Autodesk Inventor part; units mm, degrees
ref_plane "YZ Plane" through (0, 0, 0) normal (1, 0, 0) x (0, 1, 0)
ref_plane "XZ Plane" through (0, 0, 0) normal (0, 1, 0) x (-1, 0, 0)
ref_plane "XY Plane" through (0, 0, 0) normal (0, 0, 1) x (1, 0, 0)
sketch "Sketch1" plane through (0, 0, 0) normal (0, 1, 0) x (-1, 0, 0)
  circle A0 centre (0, 0) radius 6
  dimension "d0" = 12
extrude "Extrusion1" add sketch "Sketch1" along normal blind 1
fillet "Fillet1" radius 0.5 1 edges at (6, 0, 0)
sketch "Sketch2" plane through (0, 1, 0) normal (0, 1, 0) x (1, 0, 0)
  circle A0 centre (0, 0) radius 0.5
  dimension "d4" = 1
extrude "Extrusion2" cut sketch "Sketch2" against normal blind 1
sketch "Sketch3" plane through (0, 1, 0) normal (0, 1, 0) x (1, 0, 0)
  circle A0 centre (0, 0) radius 0.5
  circle A1 centre (0, 0) radius 5
  circle A2 centre (0, 0) radius 4
  dimension "d7" = 10
  dimension "d8" = 8
extrude "Extrusion3" add sketch "Sketch3" along normal blind 3 contours A1
chamfer "Chamfer1" distance 0.75 distance2 1.5 1 edges at (-4, 4, 0) measured on face at (4.5795, 4, 0.7179)
fillet "Fillet2" radius 0.2 1 edges at (-4.75, 4, 0)
fillet "Fillet3" radius 0.5 1 edges at (-4, 2.5, 0)
properties part number "tale"
Design review of the part built by this model. Coordinates are the model's own, in mm. Coordinates: 2 decimals unless noted, no trailing zeros. Write each loop counter-clockwise with the first axis right and the second up, starting at its lowest first coordinate (ties: lowest second). Pieces come first, ordered by that corner, then holes.
1) Mouldability with a two-part tool opening along X and no side actions: class faces 1 (the cylindrical face through (-0.108, 0.507, 0.488)), 2 (the flat face through (0, 0, -1)), 3 (the cylindrical face through (5.994, 0.746, -0.264)), 4 (the flat face through (0, 1, -1)) as +X half, -X half, draft (parallel to the pull), parting line (faces both ways), or undercut.
2) Add section A-A (y = 1.25). Write out the cut boundary in (x, z), plus the area to 3 significant figures.
3) To check wall thickness, follow L1, parallel to X at y = 1.45, z = 0; L2, parallel to Y at x = 4.5, z = 2.5. State the ranges of each line that lie inside material, in increasing order.
4) Insertion check: pin 1 (1.5 mm diameter, centred on y = 2, z = -1.5, fed in from -X); pin 2 (7 mm diameter, centred on x = 0, z = 0, fed in from +Y). Each pin has a flat end and moves straight along its axis. Give the tip position at first contact, or say it passes through.
Check result:
1. face 1: undercut
1. face 2: draft
1. face 3: parting line
1. face 4: undercut
2. outline: circle Ø10 at (0, 0); hole circle Ø8 at (0, 0)
2. area: 28.3 mm2
3. L1: x = -5 to -4, 4 to 5
3. L2: y = 0 to 1
4. pin 1: stops at x = -4.94
4. pin 2: stops at y = 1
